For this review, take the finished solid that the model builds, in its own axes (mm). Face numbers are marked on the shaded views. Coordinates: 2 decimals unless noted, no trailing zeros. Write each loop counter-clockwise with the first axis right and the second up, starting at its lowest first coordinate (ties: lowest second). Pieces come first, ordered by that corner, then holes. Notation, with made-up numbers: (3.25, 39) - (7.25, 39) arc R23 ccw to (7.25, 61) - close; hole circle Ø5 at (12.25, -38). An arc over 180 degrees is marked (long way). Use one line per item in the form item = value. Start each with the question number.
1) We need section D-D (y = -5). Give the boundary of the cut face in (x, z), plus the area to 3 significant figures.
2) We need section A-A (x = -5). Give the boundary of the cut face in (y, z).
3) For L1, parallel to Y at x = 8.25, z = 0; L2, parallel to Z at x = -9.25, y = 0; L3, parallel to Y at x = 14, z = 0, list the stretches that pass through material, from the lowest coordinate up. Write a range as from..to.
4) We need section B-B (y = 0). Give the boundary of the cut face in (x, z), plus the area to 3 significant figures.
5) Mouldability with a two-part tool opening along Y and no side actions: class the marked faces 1, 2, 3 and 4 as pulls with the +Y half, pulls with the -Y half, needs draft (parallel to the pull), parting line crosses it, or undercut.
6) Insertion check: P1, Ø1, axis at x = 7.5, y = 2, coming from the -Z side; P2, Ø4, axis at y = -1.5, z = 0.5, coming from the -X side; P3, Ø2, axis at x = -15, y = 3.5, coming from the +Z side. Each pin has a flat end and moves straight along its axis. Give the tip position at first contact, or say it passes through.
7) We need section C-C (x = 8). Give the boundary of the cut face in (y, z).
```python
from build123d import *

# Parameters (mm, degrees)
EXTRUDE_1_DEPTH      = 18
EXTRUDE_1_DEPTH_BACK = 20
SKETCH_1_R           = 6
SKETCH_3_R           = 3.1
CUT_EXTRUDE_1_DEPTH  = 16
SKETCH_4_R           = 4.1
CUT_EXTRUDE_2_DEPTH  = 20
EXTRUDE_START        = 12
EXTRUDE_2_DEPTH      = 12
EXTRUDE_START_2      = 15
EXTRUDE_3_DEPTH      = 15
CHAMFER_1_SIZE       = 0.4
CHAMFER_2_SIZE       = 0.5
EXTRUDE_4_REACH      = 40.936
FILLET_1_R           = 0.3


with BuildPart() as part:
    # 草图1 → 凸台-拉伸1 (new, two sides: drawn at the far end of the back side and taken through both)
    with BuildSketch(Plane(origin=(0, 0, 0), x_dir=(0, 0, -1), z_dir=(1, 0, 0)).offset(-EXTRUDE_1_DEPTH_BACK)):
        Circle(SKETCH_1_R)
    extrude(amount=EXTRUDE_1_DEPTH + EXTRUDE_1_DEPTH_BACK)

    # 草图3 → 切除-拉伸1 (cut)
    with BuildSketch(Plane(origin=(18, 0, 0), x_dir=(0, 0, -1), z_dir=(1, 0, 0))):
        Circle(SKETCH_3_R)
    extrude(amount=-CUT_EXTRUDE_1_DEPTH, mode=Mode.SUBTRACT)

    # 草图4 → 切除-拉伸2 (cut)
    with BuildSketch(Plane.ZY.offset(20)):
        Circle(SKETCH_4_R)
    extrude(amount=-CUT_EXTRUDE_2_DEPTH, mode=Mode.SUBTRACT)

    # 草图5 → 凸台-拉伸2 (add)
    with BuildSketch(Plane(origin=(2, 0, 0), x_dir=(0, 0, -1), z_dir=(1, 0, 0)).offset(EXTRUDE_START)):
        with BuildLine():
            Line((-1.688194302, 2.6), (1.688194302, 2.6))
            ThreePointArc((1.688194302, 2.6), (0, 3.1), (-1.688194302, 2.6))
        make_face()
    extrude(amount=-EXTRUDE_2_DEPTH)

    # 草图6 → 凸台-拉伸3 (add)
    with BuildSketch(Plane.ZY.offset(EXTRUDE_START_2)):
        with BuildLine():
            Line((-1.748205844, 3.708608408), (2.169358352, 3.479063716))
            ThreePointArc((2.169358352, 3.479063716), (0.239822956, 4.09297996), (-1.748205844, 3.708608408))
        make_face()
    extrude(amount=-EXTRUDE_3_DEPTH)

    # 倒角1
    chamfer_1_edges = [part.edges().sort_by_distance(p)[0] for p in [
        (-20, 0, -4.1),
        (18, 0, 3.1),
    ]]
    chamfer(chamfer_1_edges, length=CHAMFER_1_SIZE)

    # 倒角2
    chamfer_2_edges = [part.edges().sort_by_distance(p)[0] for p in [
        (-15, 3.593836062, 0.210576254),
        (14, 2.6, 0),
    ]]
    chamfer(chamfer_2_edges, length=CHAMFER_2_SIZE - 0.0001)  # a hair under: the kernel refuses the full size

    # 凸台-拉伸4: up to this face of the body (flat: up to its plane)
    extrude_4_end = Plane(part.part.faces().sort_by_distance((-20, 0, -4.669705627))[0])
    # 草图7 → 凸台-拉伸4 (add, up to the picked face)
    with BuildSketch(Plane(origin=(18, 0, 0), x_dir=(0, 0, -1), z_dir=(1, 0, 0)), mode=Mode.PRIVATE) as extrude_4_sk1:
        with BuildLine():
            Line((-1.144552314, 6.5), (-1.144552314, 4))
            Line((-1.144552314, 4), (1.144552314, 4))
            Line((1.144552314, 4), (1.144552314, 6.5))
            ThreePointArc((1.144552314, 6.5), (0, 6.6), (-1.144552314, 6.5))
        make_face()
    extrude_4_tool1 = split(extrude(extrude_4_sk1.sketch, amount=-EXTRUDE_4_REACH, mode=Mode.PRIVATE), bisect_by=extrude_4_end, keep=Keep.BOTH, mode=Mode.PRIVATE)
    add(extrude_4_tool1.solids().sort_by(Axis((18, 5.283557, 0), (-1, 0, 0)))[0])

    # 圆角1
    fillet_1_edges = [part.edges().sort_by_distance(p)[0] for p in [
        (-1, 5.889821729, -1.144552314),
        (-1, 6.5, -1.144552314),
        (-1, 5.889821729, 1.144552314),
        (-1, 6.5, 1.144552314),
    ]]
    fillet(fillet_1_edges, radius=FILLET_1_R)


solid = part.part
```
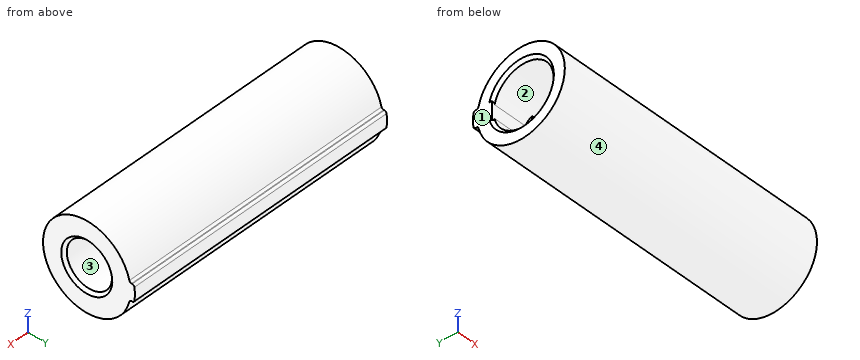
Determined:
q1.outline = (-20, -3.32) - (18, -3.32) - (18, 3.32) - (-20, 3.32) - close
q1.area = 252 mm²
q2.outline = (5.84, -1.38) arc R0.3 cw to (6.13, -1.14) - (6.24, -1.14) arc R0.3 ccw to (6.54, -0.88) arc R6.6 ccw to (6.54, 0.88) arc R0.3 ccw to (6.24, 1.14) - (6.13, 1.14) arc R0.3 cw to (5.84, 1.38) arc R6 ccw (long way) to start; hole (3.48, 2.17) arc R4.1 ccw (long way) to (3.71, -1.75) - close
q3.L1 = -6..-3.1, 2.6..6.6
q3.L2 = -6..-4.1, 4.1..6
q3.L3 = -6..-3.1, 3.1..6.6
q4.outline = (-20, -6) - (18, -6) - (18, -3.5) - (17.6, -3.1) - (2, -3.1) - (2, 3.1) - (17.6, 3.1) - (18, 3.5) - (18, 6) - (-20, 6) - (-20, 4.5) - (-19.6, 4.1) - (0, 4.1) - (0, -4.1) - (-19.6, -4.1) - (-20, -4.5) - close
q4.area = 192 mm²
q5.face_1 = needs draft
q5.face_2 = undercut
q5.face_3 = undercut
q5.face_4 = parting line crosses it
q6.P1 = -5.81
q6.P2 = 0
q6.P3 = 5.45
q7.outline = (5.84, -1.38) arc R0.3 cw to (6.13, -1.14) - (6.24, -1.14) arc R0.3 ccw to (6.54, -0.88) arc R6.6 ccw to (6.54, 0.88) arc R0.3 ccw to (6.24, 1.14) - (6.13, 1.14) arc R0.3 cw to (5.84, 1.38) arc R6 ccw (long way) to start; hole (2.6, -1.69) - (2.6, 1.69) arc R3.1 ccw (long way) to start
